Geometry: see drawing. Coordinates: mm, zero at the bounding-box minimum. A direction names the side the tool comes from. Give positions to 0.01 mm unless a question says otherwise; leave off trailing zeros. Loops run counter-clockwise (first coordinate to the right, second up) from the corner with the lowest first, then second, coordinate; pieces in that order, holes last. Notation, with made-up numbers: M 40,31 L 55,31 A31 cw 55,70 Z; hole C -36,42.5 d4. An arc over 180 degrees is marked long. Answer in a Markdown table with one row per item.
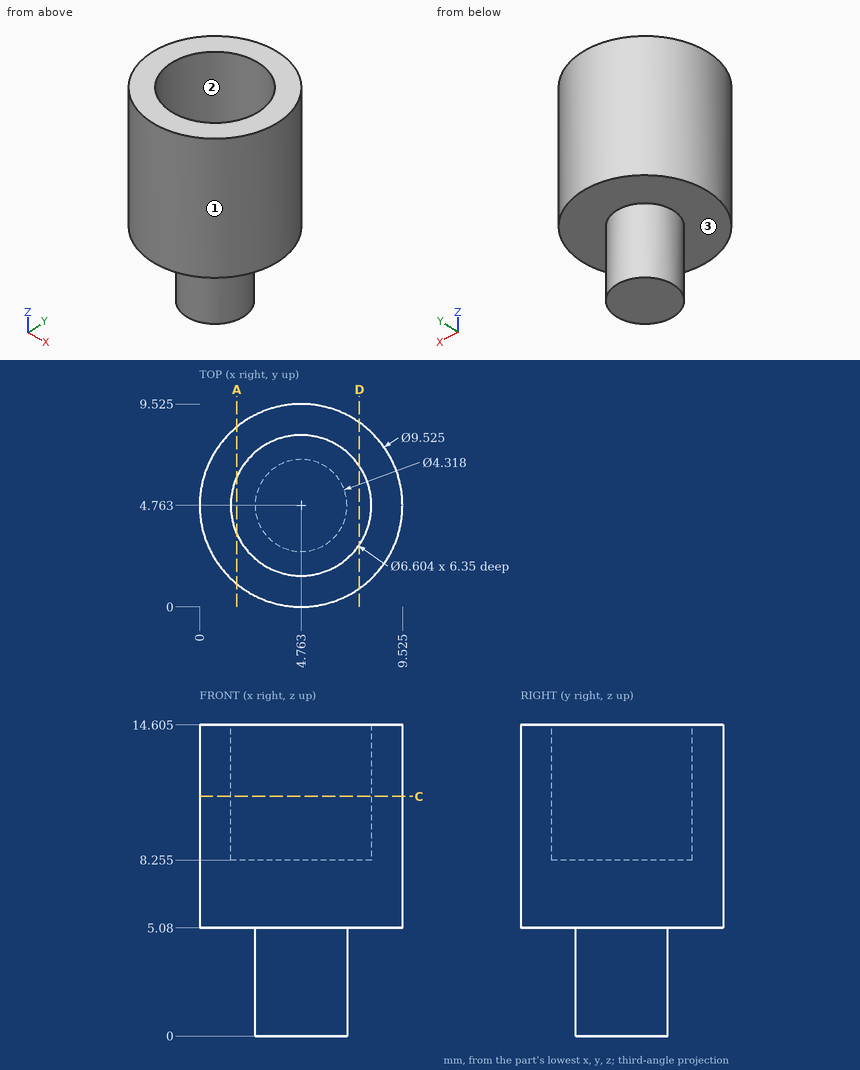
1) Section C-C, the plane z = 11.25. Return loops of the section in (x, y) (1 decimal).
Reply:
| item | result |
|---|---|
| outline | C 4.8,4.8 d9.5; hole C 4.8,4.8 d6.6 |
2) Section A-A, the plane x = 1.75. Return loops of the section in (y, z) (1 decimal), then the cut area to 3 significant figures.
Reply:
| item | result |
|---|---|
| outline | M 1.1,5.1 L 8.5,5.1 L 8.5,14.6 L 6.1,14.6 L 6.1,8.3 L 3.4,8.3 L 3.4,14.6 L 1.1,14.6 Z |
| area | 53.1 mm² |
3) Pin query (flat end, axial travel): pin 1 Ø3 at (y, z) = (6, 10.5) entering from +X (1 decimal); pin 2 Ø1.5 at (x, y) = (5, 7) entering from +Z (1 decimal). Return the tip coordinate at first contact, or that it passes through.
Reply:
| item | result |
|---|---|
| pin 1 | stops at x = 9.5 |
| pin 2 | stops at z = 8.3 |
4) Material intervals for L1, parallel to Z at x = 3.5, y = 5.25 (1 decimal); L2, parallel to Y at x = 2.5, z = 10 (1 decimal); L3, parallel to Z at x = 7.25, y = 2.75 (1 decimal), sorted ascending.
Reply:
| item | result |
|---|---|
| L1 | z = 0 to 8.3 |
| L2 | y = 0.6 to 2.4, 7.2 to 9 |
| L3 | z = 5.1 to 8.3 |
5) Set-up query: the marked faces 1, 2 and 3. Return all of +Z, -Z, +X, -X, +Y, -Y with unobstructed straight access to the full face (end or side cutting, diameter ignored); none if empty.
Reply:
| item | result |
|---|---|
| face 1 | +Z, -Z |
| face 2 | +Z |
| face 3 | -Z |
6) Section D-D, the plane x = 7.5. Return loops of the section in (y, z) (1 decimal).
Reply:
| item | result |
|---|---|
| outline | M 0.9,5.1 L 8.7,5.1 L 8.7,14.6 L 6.6,14.6 L 6.6,8.3 L 2.9,8.3 L 2.9,14.6 L 0.9,14.6 Z |
